Drawing for the job (mm, zero at the part's lowest x, y, z). A direction names the side the tool comes from. Coordinates: 2 decimals unless noted, no trailing zeros. Write each loop counter-clockwise with the first axis right and the second up, starting at its lowest first coordinate (ties: lowest second). Pieces come first, ordered by that corner, then holes. Notation, with made-up numbers: M 0,26.5 L 6,26.5 A27 ccw 6,49.5 Z; hole C 56.5,83.25 d7. An arc over 180 degrees is marked long. Use a Markdown table: item, result. Add a question column.
Q1. Slice it at B-B on x = 28.5. Write the cut outline in (y, z), then the cut area to 3 significant figures.
Q2. Slice it at D-D on x = 36.5. Write the cut outline in (y, z) (3 decimals).
Q3. Slice it at C-C on z = 8.5. Write the cut outline in (x, y) (3 decimals).
Q4. Pin check, flat tips, straight feed: pin 1 Ø6 at (x, y) = (21, 5) entering from -Z; pin 2 Ø3.5 at (x, y) = (5.5, 36.5) entering from -Z. Stop position of each tip, or through.
Q5. Slice it at A-A on y = 36.5. Write the cut outline in (x, z) (3 decimals), then the cut area to 3 significant figures.
Q6. Tool access for the marked faces 5 and 6: list every direction of +Z, -Z, +X, -X, +Y, -Y with a clear straight run to the whole face (end or side of a thin tool).
Q7. Wall check: L1, parallel to Y at x = 36.5, z = 6.75 (3 decimals); L2, parallel to X at y = 36.5, z = 4.5 (3 decimals); L3, parallel to Y at x = 30, z = 4.5. Give the ranges that are in metal, low to high. Write a range as from..to.
Q8. Mould opens along Y. For the marked faces 1, 2, 3 and 4 say: released by +Y, released by -Y, zero draft, split by the parting line, or undercut.
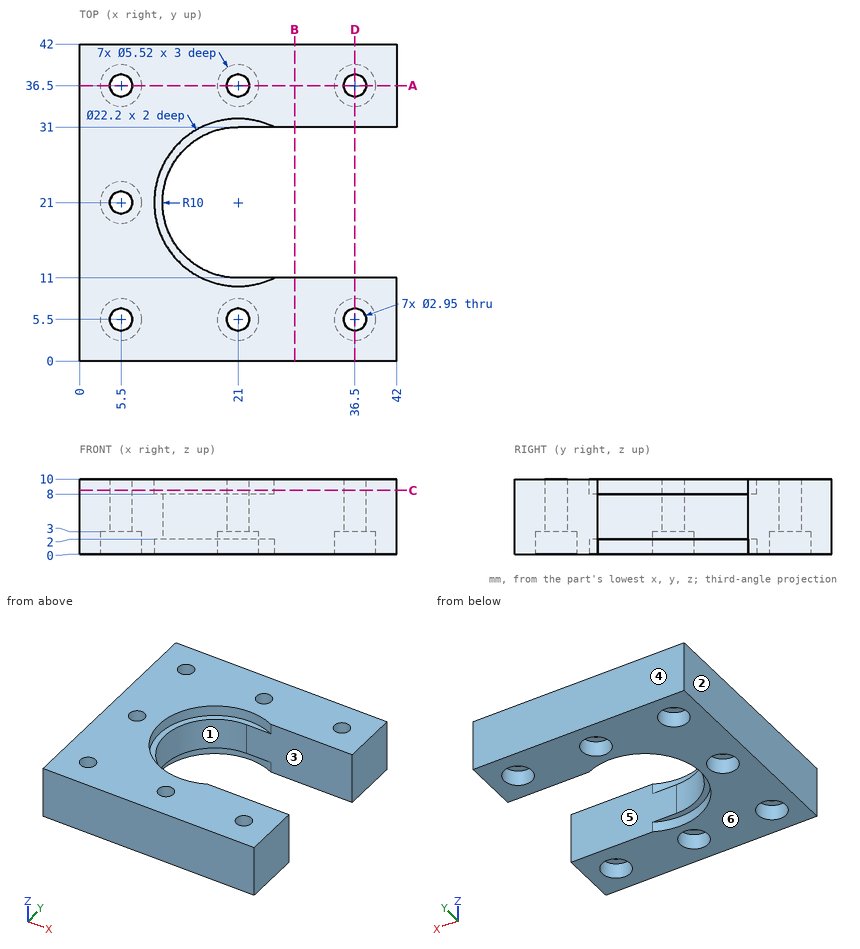
Recorded:
| question | item | result |
|---|---|---|
| 1 | outline | M 0,0 L 11,0 L 11,10 L 0,10 Z; M 31,0 L 42,0 L 42,10 L 31,10 Z |
| 1 | area | 220 mm² |
| 2 | outline | M 0,0 L 2.74,0 L 2.74,3 L 4.025,3 L 4.025,10 L 0,10 Z; M 6.975,3 L 8.26,3 L 8.26,0 L 11,0 L 11,10 L 6.975,10 Z; M 31,0 L 33.74,0 L 33.74,3 L 35.025,3 L 35.025,10 L 31,10 Z; M 37.975,3 L 39.26,3 L 39.26,0 L 42,0 L 42,10 L 37.975,10 Z |
| 3 | outline | M 0,0 L 42,0 L 42,11 L 25.818,11 A11.1 cw long 25.818,31 L 42,31 L 42,42 L 0,42 Z; hole C 5.5,5.5 d2.95; hole C 5.5,21 d2.95; hole C 5.5,36.5 d2.95; hole C 21,5.5 d2.95; hole C 21,36.5 d2.95; hole C 36.5,5.5 d2.95; hole C 36.5,36.5 d2.95 |
| 4 | pin 1 | z = 0 |
| 4 | pin 2 | z = 3 |
| 5 | outline | M 0,0 L 2.74,0 L 2.74,3 L 4.025,3 L 4.025,10 L 0,10 Z; M 6.975,3 L 8.26,3 L 8.26,0 L 18.24,0 L 18.24,3 L 19.525,3 L 19.525,10 L 6.975,10 Z; M 22.475,3 L 23.76,3 L 23.76,0 L 33.74,0 L 33.74,3 L 35.025,3 L 35.025,10 L 22.475,10 Z; M 37.975,3 L 39.26,3 L 39.26,0 L 42,0 L 42,10 L 37.975,10 Z |
| 5 | area | 308 mm² |
| 6 | face 5 | +Z, -Z, +X |
| 6 | face 6 | -Z, +X, -X, +Y, -Y |
| 7 | L1 | 0..4.025, 6.975..11, 31..35.025, 37.975..42 |
| 7 | L2 | 0..4.025, 6.975..19.525, 22.475..35.025, 37.975..42 |
| 7 | L3 | 0..11, 31..42 |
| 8 | face 1 | undercut |
| 8 | face 2 | zero draft |
| 8 | face 3 | undercut |
| 8 | face 4 | released by +Y |
